```python
from build123d import *

# Parameters (mm, degrees)
F1_DEPTH = 2
F2_R     = 4.5
F3_DEPTH = 0.5


with BuildPart() as f1:
    # F0 (on Top) → F1 (new body)
    with BuildSketch(Plane.XY):
        with BuildLine():
            ThreePointArc((-49.731933, -6), (-45.489292, -4.242641), (-43.731933, 0))
            ThreePointArc((-43.731933, 0), (-45.489292, 4.242641), (-49.731933, 6))
            ThreePointArc((-49.731933, 6), (-55.731933, 0), (-49.731933, -6))
        make_face()
        with BuildLine():
            ThreePointArc((-49.731933, 6), (-45.489292, 4.242641), (-43.731933, 0))
            ThreePointArc((-43.731933, 0), (-45.489292, -4.242641), (-49.731933, -6))
            Line((-49.731933, -6), (-26.731933, -6))
            ThreePointArc((-26.731933, -6), (-32.731933, 0), (-26.731933, 6))
            Line((-26.731933, 6), (-49.731933, 6))
        make_face()
        with BuildLine():
            ThreePointArc((-20.731933, 0), (-22.489292, 4.242641), (-26.731933, 6))
            ThreePointArc((-26.731933, 6), (-32.731933, 0), (-26.731933, -6))
            ThreePointArc((-26.731933, -6), (-22.489292, -4.242641), (-20.731933, 0))
        make_face()
    extrude(amount=F1_DEPTH)

    # F2 (on face) → F3 (cut)
    with BuildSketch(Plane.XY.offset(2)):
        with Locations((-49.731933, 0)):
            Circle(F2_R)
        with Locations((-26.731933, 0)):
            Circle(F2_R)
    extrude(amount=-F3_DEPTH, mode=Mode.SUBTRACT)


solid = f1.part
```
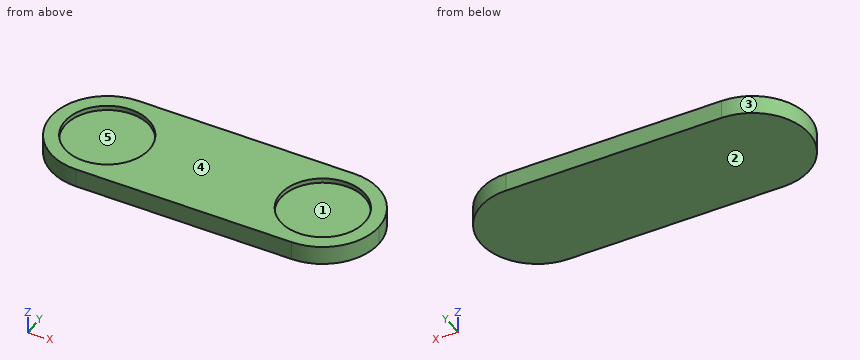
Design review of the part built by this model. Coordinates are the model's own, in mm. Face numbers are marked on the shaded views. A direction names the side the tool comes from. Coordinates: 2 decimals unless noted, no trailing zeros. Loops run counter-clockwise (first coordinate to the right, second up) from the corner with the lowest first, then second, coordinate; pieces in that order, holes last. Notation, with made-up numbers: (25.5, -23.5) -> (70.5, -23.5) arc R26 cw to (70.5, -6.5) -> close; hole circle Ø9 at (11, 6.5). An arc over 180 degrees is marked (long way). Answer as a JSON object with one key per item and string values.
Q1. The part is to be moulded in two halves that separate along Y. For the marked faces 1, 2 and 3, say which applies: +Y half, -Y half, draft (parallel to the pull), parting line (faces both ways), or undercut.
Answer block:
{"face 1": "undercut", "face 2": "draft", "face 3": "parting line"}
Q2. Tool access review of the marked faces 4 and 5: name each direction out of +Z, -Z, +X, -X, +Y, -Y from which nothing blocks a thin tool from reaching the whole face with its end or side.
Answer block:
{"face 4": "+Z, +X, -X, +Y, -Y", "face 5": "+Z"}
Q3. Take a section at A-A on z = 1.1. Give the boundary of the cut face in (x, y).
Answer block:
{"outline": "(-49.73, -6) -> (-26.73, -6) arc R6 ccw to (-20.73, 0) arc R6 ccw to (-26.73, 6) -> (-49.73, 6) arc R6 ccw to start"}
Q4. Take a section at B-B on x = -30.5. Give the boundary of the cut face in (y, z).
Answer block:
{"outline": "(-6, 0) -> (6, 0) -> (6, 2) -> (2.46, 2) -> (2.46, 1.5) -> (-2.46, 1.5) -> (-2.46, 2) -> (-6, 2) -> close"}
Q5. Take a section at C-C on y = -3. Give the boundary of the cut face in (x, z), plus the area to 3 significant figures.
Answer block:
{"outline": "(-54.93, 0) -> (-21.54, 0) -> (-21.54, 2) -> (-23.38, 2) -> (-23.38, 1.5) -> (-30.09, 1.5) -> (-30.09, 2) -> (-46.38, 2) -> (-46.38, 1.5) -> (-53.09, 1.5) -> (-53.09, 2) -> (-54.93, 2) -> close", "area": "60.1 mm^2"}
Q6. Take a section at D-D on x = -52. Give the boundary of the cut face in (y, z).
Answer block:
{"outline": "(-5.55, 0) -> (5.55, 0) -> (5.55, 2) -> (3.89, 2) -> (3.89, 1.5) -> (-3.89, 1.5) -> (-3.89, 2) -> (-5.55, 2) -> close"}
Q7. Clearance check with a flat-ended pin moving along its axis: pin 1 Ø4.5 at (x, y) = (-48.5, 0) entering from +Z. State where the tip first meets the part, or that it passes through.
Answer block:
{"pin 1": "stops at z = 1.5"}
Q8. To check wall thickness, follow L1, parallel to Z at x = -52, y = 1; L2, parallel to X at y = 0.25, z = 0.6; L3, parallel to X at y = 4.5, z = 0.3. State the ranges of each line that lie inside material, in increasing order.
Answer block:
{"L1": "z = 0 to 1.5", "L2": "x = -55.73 to -20.74", "L3": "x = -53.7 to -22.76"}
